from build123d import *

# Parameters (mm, degrees)
SKETCH_1_W          = 25
SKETCH_1_H          = 25
EXTRUDE_1_DEPTH     = 44.284173786
SKETCH_2_R          = 3
CUT_EXTRUDE_1_DEPTH = 36.406845426
SKETCH_4_W          = 25
SKETCH_4_H          = 12
CUT_EXTRUDE_2_DEPTH = 18.639834826
CUT_EXTRUDE_3_DEPTH = 40


with BuildPart() as part:
    # 스케치1 → 보스-돌출1 (new body)
    with BuildSketch(Plane.XY):
        Rectangle(SKETCH_1_W, SKETCH_1_H)
    extrude(amount=EXTRUDE_1_DEPTH)

    # 스케치2 → 컷-돌출1 (cut)
    with BuildSketch(Plane(origin=(0, 12.5, 0), x_dir=(1, 0, 0), z_dir=(0, 1, 0))):
        with Locations(Location((0, -39.284173786, 0), (0, 0, 270))):
            Circle(SKETCH_2_R)
    extrude(amount=-CUT_EXTRUDE_1_DEPTH, mode=Mode.SUBTRACT)

    # 스케치4 → 컷-돌출2 (cut)
    with BuildSketch(Plane.XY.offset(44.284173786)):
        Rectangle(SKETCH_4_W, SKETCH_4_H)
    extrude(amount=-CUT_EXTRUDE_2_DEPTH, mode=Mode.SUBTRACT)

    # 스케치5 → 컷-돌출3 (cut)
    with BuildSketch(Plane(origin=(0, 12.5, 0), x_dir=(1, 0, 0), z_dir=(0, 1, 0))):
        with BuildLine():
            Line((-47.02485921, -52.228316923), (5.705393133, 41.461873578))
            Line((5.705393133, 41.461873578), (28.83172343, -24.155832398))
            Line((28.83172343, -24.155832398), (12.5, -44.284173786))
            add(Edge.make_bspline(
                [(0, 0), (17.942606177, -19.069541042), (12.5, -44.284173786)],
                knots=[0, 0, 0, 1, 1, 1], degree=2))
            add(Edge.make_bspline(
                [(0, 0), (5.442606177, -25.214632744), (-12.5, -44.284173786)],
                knots=[0, 0, 0, 1, 1, 1], degree=2))
            Line((-12.5, -44.284173786), (-47.02485921, -52.228316923))
        make_face()
    extrude(amount=-CUT_EXTRUDE_3_DEPTH, mode=Mode.SUBTRACT)


solid = part.part
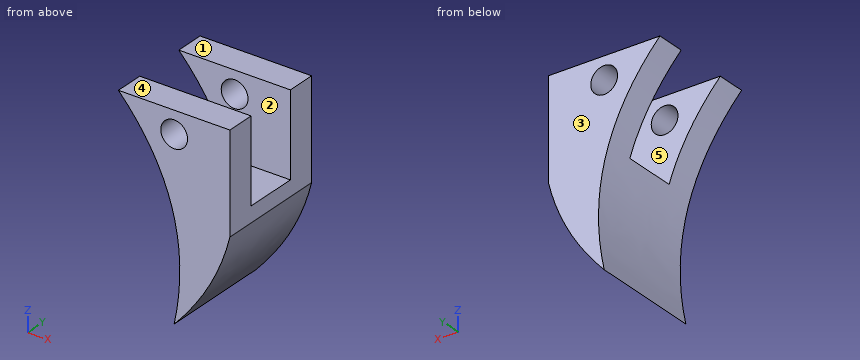
Can you work these out from the model? Positions are in its coordinate system, mm. Face numbers are marked on the shaded views. A direction names the side the tool comes from. Coordinates: 2 decimals unless noted, no trailing zeros. Answer as a JSON object with one key per item and string values. Group by question number.
Q1. We'd pull the mould along Y, two halves only. Please class the marked faces 1, 2 and 3: +Y half, -Y half, draft (parallel to the pull), parting line (faces both ways), or undercut.
Q2. On a 3-axis mill with a long thin cutter (end or side, diameter ignored), from which of +Z, -Z, +X, -X, +Y, -Y can I reach the whole of each face in a straight line? I mean the marked faces 4 and 5. Say none if no direction works.
Q3. Will these pins go through, and if not, where does the flat tip stop? P1, Ø3.5, axis at x = 8, y = -1, coming from the +Z side; P2, Ø2, axis at x = -2.5, y = 2, coming from the +Z side; P3, Ø5, axis at y = -9, z = 9, coming from the -X side; P4, Ø3, axis at y = -4.5, z = 16.5, coming from the -X side.
Q4. I need wall thicknesses on line 1 (Y direction, x = 3, z = 29); line 2 (X direction, y = 9.5, z = 17.5); line 3 (Z direction, x = -2, y = -8.75). Which ranges of each line are inside material? Lowest first, please. Write a range as from..to.
Determined:
{
 "1": {"face 1": "draft", "face 2": "undercut", "face 3": "+Y half"},
 "2": {"face 4": "+Z, +X, -X, +Y, -Y", "face 5": "+Z, +X, -X"},
 "3": {"P1": "stops at z = 25.64", "P2": "passes through", "P3": "stops at x = 1.02", "P4": "stops at x = 0.8"},
 "4": {"line 1": "y = -12.5..-6, 6..12.5", "line 2": "x = 0.87..11.09", "line 3": "z = 28.32..37.05, 41.52..44.28"}
}
